Part model, mm, in its own coordinate system. A direction names the side the tool comes from. Give positions to 0.01 mm unless a question says otherwise; leave off trailing zeros. Loops run counter-clockwise (first coordinate to the right, second up) from the corner with the lowest first, then second, coordinate; pieces in that order, holes last. Notation, with made-up numbers: M 52,70 L 83,70 A13 cw 83,84 Z; hole C -11,89.25 d5. An arc over 180 degrees is marked long. Answer in a Markdown table with one row per item.
from build123d import *

# Parameters (mm, degrees)
F1_DEPTH = 15
F2_R     = 1


with BuildPart() as f1:
    # F0 (on Top) → F1 (new body)
    with BuildSketch(Plane.XY):
        Polygon((5.65, -6.02132), (5.65, 9.5), (-5.65, 9.5), (-5.65, -6.02132), (-2.27132, -9.4), (2.27132, -9.4), align=None)
        Polygon((-4.15, 8), (4.15, 8), (4.15, -5.4), (1.65, -7.9), (-1.65, -7.9), (-4.15, -5.4), align=None, mode=Mode.SUBTRACT)
    extrude(amount=F1_DEPTH)

    # F2
    f2_edges = [f1.edges().sort_by_distance(p)[0] for p in [
        (-5.65, 9.5, 7.5),
        (5.65, 9.5, 7.5),
        (5.65, -6.02132, 7.5),
        (2.27132, -9.4, 7.5),
        (-2.27132, -9.4, 7.5),
        (-5.65, -6.02132, 7.5),
    ]]
    fillet(f2_edges, radius=F2_R)


solid = f1.part
(1) Saw through at C-C (z = 13). Write the cut outline in (x, y), plus the area to 3 significant figures.
Recorded:
| item | result |
|---|---|
| outline | M -5.65,-5.61 A1 ccw -5.36,-6.31 L -2.56,-9.11 A1 ccw -1.86,-9.4 L 1.86,-9.4 A1 ccw 2.56,-9.11 L 5.36,-6.31 A1 ccw 5.65,-5.61 L 5.65,8.5 A1 ccw 4.65,9.5 L -4.65,9.5 A1 ccw -5.65,8.5 Z; hole M -4.15,-5.4 L -1.65,-7.9 L 1.65,-7.9 L 4.15,-5.4 L 4.15,8 L -4.15,8 Z |
| area | 75.9 mm^2 |
(2) Saw through at A-A (x = 0.5). Write the cut outline in (y, z).
Recorded:
| item | result |
|---|---|
| outline | M -9.4,0 L -7.9,0 L -7.9,15 L -9.4,15 Z; M 8,0 L 9.5,0 L 9.5,15 L 8,15 Z |
(3) Saw through at D-D (x = 5). Write the cut outline in (y, z), plus the area to 3 significant figures.
Recorded:
| item | result |
|---|---|
| outline | M -6.67,0 L 9.44,0 L 9.44,15 L -6.67,15 Z |
| area | 242 mm^2 |
(4) Which spindle directions (+Z, -Z, +X, -X, +Y, -Y) get a long thin tool onto all of the face, cutting with end or side? Do faces 4 (the face through (-5.65, 2, 7)), 5 (the face through (0, -7.9, 7)). Say none if no direction does.
Recorded:
| item | result |
|---|---|
| face 4 | +Z, -Z, -X, +Y, -Y |
| face 5 | +Z, -Z |
(5) Pull direction Y, two halves, no side cores. Call faces 1 (the face through (0, 9.5, 7)), 2 (the face through (0, 8, 7)), 3 (the face through (-5, 0, 0)): +Y half, -Y half, draft (parallel to the pull), parting line (faces both ways), or undercut.
Recorded:
| item | result |
|---|---|
| face 1 | +Y half |
| face 2 | undercut |
| face 3 | draft |
(6) Pin check, flat tip, straight feed: pin 1 Ø1.5 at (x, y) = (2, 6) entering from -Z. Stop position of the tip, or through.
Recorded:
| item | result |
|---|---|
| pin 1 | passes through |
(7) Drill centre lines: line 1 along X through (y, z) = (5, 2.25); line 2 along Y through (x, z) = (0.5, 13); line 3 along X through (y, z) = (-6, 3). Where is each one in solid material? Low to high.
Recorded:
| item | result |
|---|---|
| line 1 | x = -5.65 to -4.15, 4.15 to 5.65 |
| line 2 | y = -9.4 to -7.9, 8 to 9.5 |
| line 3 | x = -5.57 to -3.55, 3.55 to 5.57 |
(8) Saw through at B-B (y = 1.5). Write the cut outline in (x, z), plus the area to 3 significant figures.
Recorded:
| item | result |
|---|---|
| outline | M -5.65,0 L -4.15,0 L -4.15,15 L -5.65,15 Z; M 4.15,0 L 5.65,0 L 5.65,15 L 4.15,15 Z |
| area | 45.0 mm^2 |
